Check sheet for the drawn part. Datum: minimum x, y, z corner. Units: mm. Round coordinates to 2 decimals unless told otherwise and drop trailing zeros. Order: outer loops, then holes, each group sorted by start corner. A loop starts at its lowest first (then second) coordinate and runs counter-clockwise, first axis right, second up. Notation, with made-up numbers: M 85,19.5 L 130,19.5 A12 cw 130,29.5 Z; hole C 87,-40 d8. An arc over 180 degrees is marked long. Answer as a JSON object with one key per item and string values. Group by question number.
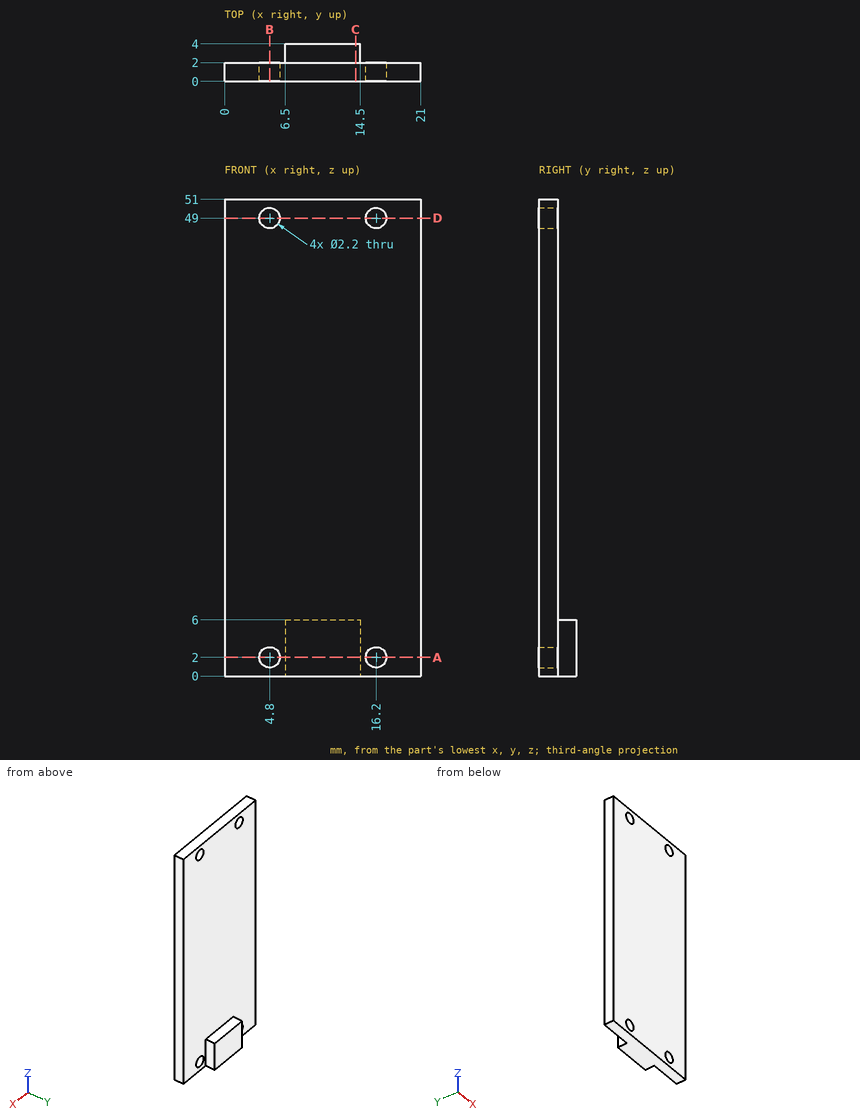
1) Sectioned sample at D-D (z = 49). Record the boundary of the cut face in (x, y), then the cut area to 3 significant figures.
2) Sectioned sample at A-A (z = 2). Record the boundary of the cut face in (x, y).
3) Go/stop test with flat-tipped pins: P1, Ø1.6, axis at y = 3.5, z = 2, coming from the +X side; P2, Ø4, axis at x = 8.5, z = 10, coming from the +Y side; P3, Ø1, axis at x = 9.5, y = 3, coming from the +Z side. Record where each tip stops, or that it passes through.
4) Sectioned sample at B-B (x = 4.8). Record the boundary of the cut face in (y, z).
5) Sectioned sample at C-C (x = 14). Record the boundary of the cut face in (y, z).
6) Thickness scan on line 1 along Z through (x, y) = (16.2, 1.05); line 2 along X through (y, z) = (1.45, 2); line 3 along Y through (x, z) = (4.25, 5.5). Record the ranges inside material, lowest first. Write a range as [from, to].
Final values:
{
 "1": {"outline": "M 0,0 L 3.7,0 L 3.7,2 L 0,2 Z; M 5.9,0 L 15.1,0 L 15.1,2 L 5.9,2 Z; M 17.3,0 L 21,0 L 21,2 L 17.3,2 Z", "area": "33.2 mm^2"},
 "2": {"outline": "M 0,0 L 3.7,0 L 3.7,2 L 0,2 Z; M 5.9,0 L 15.1,0 L 15.1,2 L 14.5,2 L 14.5,4 L 6.5,4 L 6.5,2 L 5.9,2 Z; M 17.3,0 L 21,0 L 21,2 L 17.3,2 Z"},
 "3": {"P1": "stops at x = 14.5", "P2": "stops at y = 2", "P3": "stops at z = 6"},
 "4": {"outline": "M 0,0 L 2,0 L 2,0.9 L 0,0.9 Z; M 0,3.1 L 2,3.1 L 2,47.9 L 0,47.9 Z; M 0,50.1 L 2,50.1 L 2,51 L 0,51 Z"},
 "5": {"outline": "M 0,0 L 4,0 L 4,6 L 2,6 L 2,51 L 0,51 Z"},
 "6": {"line 1": "z = [0, 0.9], [3.1, 47.9], [50.1, 51]", "line 2": "x = [0, 3.7], [5.9, 15.1], [17.3, 21]", "line 3": "y = [0, 2]"}
}
